from build123d import *

# Parameters (mm, degrees)
SKETCH1_W           = 19.05
SKETCH1_H           = 50.8
BOSS_EXTRUDE1_DEPTH = 6.35
SKETCH2_W           = 4.572
SKETCH2_H           = 10.16
CUT_EXTRUDE1_DEPTH  = 7.35
SKETCH3_R           = 1.5875
CUT_EXTRUDE2_DEPTH  = 7.35


with BuildPart() as part:
    # Sketch1 → Boss-Extrude1 (new body)
    with BuildSketch(Plane.XY):
        with Locations((9.525, 25.4)):
            Rectangle(SKETCH1_W, SKETCH1_H)
    extrude(amount=BOSS_EXTRUDE1_DEPTH)

    # Sketch2 → Cut-Extrude1 (cut, through all)
    with BuildSketch(Plane.XY.offset(6.35)):
        with Locations((16.764, 45.72)):
            Rectangle(SKETCH2_W, SKETCH2_H)
        with Locations((16.764, 25.4)):
            Rectangle(SKETCH2_W, SKETCH2_H)
        with Locations((16.764, 5.08)):
            Rectangle(SKETCH2_W, SKETCH2_H)
    extrude(amount=-CUT_EXTRUDE1_DEPTH, mode=Mode.SUBTRACT)

    # Sketch3 → Cut-Extrude2 (cut, through all)
    with BuildSketch(Plane.XY.offset(6.35)):
        with Locations((7.239, 38.1)):
            Circle(SKETCH3_R)
        with Locations((7.239, 25.4)):
            Circle(SKETCH3_R)
        with Locations((7.239, 12.7)):
            Circle(SKETCH3_R)
    extrude(amount=-CUT_EXTRUDE2_DEPTH, mode=Mode.SUBTRACT)


solid = part.part
The model under review builds one solid part; all positions refer to its coordinate system, in mm. A direction names the side the tool comes from. Round coordinates to 2 decimals unless told otherwise and drop trailing zeros. Loops run counter-clockwise (first coordinate to the right, second up) from the corner with the lowest first, then second, coordinate; pieces in that order, holes last. Notation, with made-up numbers: (31, 25.25) - (48, 25.25) arc R10 ccw to (48, 41.25) - close; hole circle Ø8 at (59.5, 67.5). An arc over 180 degrees is marked (long way). Use CSV: the item, a comma, the result in double quotes.
(1) Take a section at A-A, the plane y = 25.4. Give the boundary of the cut face in (x, z).
Working result:
outline,"(0, 0) - (5.65, 0) - (5.65, 6.35) - (0, 6.35) - close; (8.83, 0) - (14.48, 0) - (14.48, 6.35) - (8.83, 6.35) - close"
(2) For line 1 (Y direction, x = 16.5, z = 1.25); line 2 (Y direction, x = 8.5, z = 3.75); line 3 (X direction, y = 23, z = 1), list the stretches that pass through material, from the lowest coordinate up.
Working result:
line 1,"y = 10.16 to 20.32, 30.48 to 40.64"
line 2,"y = 0 to 11.74, 13.66 to 24.44, 26.36 to 37.14, 39.06 to 50.8"
line 3,"x = 0 to 14.48"
(3) The part is to be moulded in two halves that separate along Y. For faces 1 (the flat face through (17, 20.32, 3)), 2 (the cylindrical face through (8.09, 26.74, 3.22)), 3 (the flat face through (9, 26, 6.35)), 4 (the flat face through (17, 10.16, 3)), say which applies: pulls with the +Y half, pulls with the -Y half, needs draft (parallel to the pull), parting line crosses it, or undercut.
Working result:
face 1,"undercut"
face 2,"undercut"
face 3,"needs draft"
face 4,"pulls with the -Y half"
(4) Take a section at B-B, the plane x = 15.75. Give the boundary of the cut face in (y, z).
Working result:
outline,"(10.16, 0) - (20.32, 0) - (20.32, 6.35) - (10.16, 6.35) - close; (30.48, 0) - (40.64, 0) - (40.64, 6.35) - (30.48, 6.35) - close"
(5) Take a section at C-C, the plane z = 4.25. State how many separate pieces and enclosed holes the cut face has, plus the area to 3 significant figures.
Working result:
separate pieces,"1"
enclosed holes,"3"
area,"805 mm^2"
(6) Machinability: for faces 5 (the flat face through (14.478, 25, 3)), 6 (the flat face through (14.478, 5, 3)), 7 (the flat face through (19.05, 35, 3)), 8 (the flat face through (7, 50.8, 3)), 9 (the flat face through (14.478, 46, 3)), which of the approach directions +Z, -Z, +X, -X, +Y, -Y give a long, thin tool a straight path to every point of the face, cutting with its end or side? Answer none if there is none.
Working result:
face 5,"+Z, -Z, +X"
face 6,"+Z, -Z, +X, -Y"
face 7,"+Z, -Z, +X, +Y, -Y"
face 8,"+Z, -Z, +X, -X, +Y"
face 9,"+Z, -Z, +X, +Y"
(7) Clearance check with flat-ended pins moving along their axes: P1, Ø1.9, axis at y = 23, z = 2, coming from the +X side; P2, Ø3.5, axis at x = 17.5, z = 1.5, coming from the -Y side; P3, Ø1.9, axis at x = 7.239, y = 38.1, coming from the +Z side; P4, Ø1.4, axis at x = 17, z = 3.5, coming from the +Y side. State where each tip first meets the part, or that it passes through.
Working result:
P1,"stops at x = 14.48"
P2,"stops at y = 10.16"
P3,"passes through"
P4,"stops at y = 40.64"
(8) Take a section at D-D, the plane x = 8. Give the boundary of the cut face in (y, z), plus the area to 3 significant figures.
Working result:
outline,"(0, 0) - (11.31, 0) - (11.31, 6.35) - (0, 6.35) - close; (14.09, 0) - (24.01, 0) - (24.01, 6.35) - (14.09, 6.35) - close; (26.79, 0) - (36.71, 0) - (36.71, 6.35) - (26.79, 6.35) - close; (39.49, 0) - (50.8, 0) - (50.8, 6.35) - (39.49, 6.35) - close"
area,"269 mm^2"
